```python
from build123d import *

# Parameters (mm, degrees)
SKETCH1_R           = 1.7907
SKETCH1_R_2         = 2.2987
BOSS_EXTRUDE1_DEPTH = 6.35
FILLET1_R           = 2.54
SKETCH2_W           = 2.54
SKETCH2_H           = 12.7
CUT_EXTRUDE1_DEPTH  = 6.35


with BuildPart() as part:
    # Sketch1 → Boss-Extrude1 (new body)
    with BuildSketch(Plane(origin=(0, 0, 0), x_dir=(1, 0, 0), z_dir=(0, 1, 0))):
        with BuildLine():
            Line((-12.7, -8.1407), (12.7, -8.1407))
            Line((12.7, -8.1407), (7.941309086, -1.7907))
            ThreePointArc((7.941309086, -1.7907), (7.76561659, 2.442579676), (5.48636952, 6.014212))
            ThreePointArc((5.48636952, 6.014212), (0, 21.3487), (-5.48636952, 6.014212))
            ThreePointArc((-5.48636952, 6.014212), (-7.76561659, 2.442579676), (-7.941309086, -1.7907))
            Line((-7.941309086, -1.7907), (-12.7, -8.1407))
        make_face()
        Circle(SKETCH1_R, mode=Mode.SUBTRACT)
        with Locations((0, 12.7)):
            Circle(SKETCH1_R_2, mode=Mode.SUBTRACT)
    extrude(amount=BOSS_EXTRUDE1_DEPTH)

    # Fillet1
    fillet1_edges = [part.edges().sort_by_distance(p)[0] for p in [
        (-7.941309086, 3.175, 1.7907),
        (-5.48636952, 3.175, -6.014212),
        (5.48636952, 3.175, -6.014212),
        (7.941309086, 3.175, 1.7907),
        (12.7, 3.175, 8.1407),
        (-12.7, 3.175, 8.1407),
    ]]
    fillet(fillet1_edges, radius=FILLET1_R)

    # Sketch2 → Cut-Extrude1 (cut)
    with BuildSketch(Plane(origin=(0, 6.35, 0), x_dir=(1, 0, 0), z_dir=(0, 1, 0))):
        with Locations((0, 12.7)):
            Rectangle(SKETCH2_W, SKETCH2_H)
    extrude(amount=-CUT_EXTRUDE1_DEPTH, mode=Mode.SUBTRACT)


solid = part.part
```
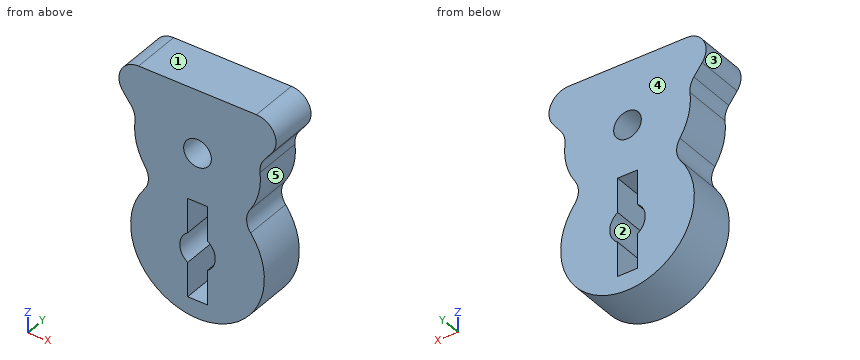
Source: CAD feature listing. Evaluate the final solid. Frame: model axes, mm. Face numbers are marked on the shaded views. A direction names the side the tool comes from. Coordinates: 2 decimals unless noted, no trailing zeros. Loops run counter-clockwise (first coordinate to the right, second up) from the corner with the lowest first, then second, coordinate; pieces in that order, holes last. Notation, with made-up numbers: (34, -22.75) -> (89, -22.75) arc R18 cw to (89, 0.25) -> close; hole circle Ø9 at (19.25, 28). An arc over 180 degrees is marked (long way). One line per item, written item: value. Start each with the question number.
Q1. Section query C-C, the plane z = -18.25. Return the cut outline in (x, y), and give its area (3 significant figures).
Q2. Section query D-D, the plane y = 5.5. Give the number of separate pieces and of enclosed holes in the cut face, and give its area (3 significant figures).
Q3. Section query A-A, the plane z = -12.7. Return the cut outline in (x, y), and give its area (3 significant figures).
Q4. Section query B-B, the plane x = 0. Return the cut outline in (y, z).
Q5. Mould query, pull axis Z, two halves, no side actions, for the marked faces 3, 4 and 5. Classes: pulls with the +Z half, pulls with the -Z half, needs draft (parallel to the pull), parting line crosses it, or undercut.
Q6. Contact query for flat-ended pins moving along their axis: P1, Ø2, axis at x = 7, y = 1, coming from the -Z side; P2, Ø2, axis at y = 5.5, z = -12, coming from the +X side; P3, Ø2, axis at y = 3, z = -9, coming from the +X side; P4, Ø2, axis at x = 0, z = 0, coming from the +Y side. Output: stop coordinate, or through.
Q7. Line query: line 1 along Z through (x, y) = (0, 4.25); line 2 along X through (y, z) = (2.5, 0); line 3 along Z through (x, y) = (-7, 5.5). Output: solid intervals per line, ascending.
Q8. Set-up query: the marked faces 1 and 2. Return all of +Z, -Z, +X, -X, +Y, -Y with unobstructed straight access to the full face (end or side cutting, diameter ignored); none if empty.
Results:
1. outline: (-6.63, 0) -> (-1.27, 0) -> (-1.27, 6.35) -> (-6.63, 6.35) -> close; (1.27, 0) -> (6.63, 0) -> (6.63, 6.35) -> (1.27, 6.35) -> close
1. area: 68.1 mm^2
2. separate pieces: 1
2. enclosed holes: 2
2. area: 411 mm^2
3. outline: (-8.65, 0) -> (-2.3, 0) -> (-2.3, 6.35) -> (-8.65, 6.35) -> close; (2.3, 0) -> (8.65, 0) -> (8.65, 6.35) -> (2.3, 6.35) -> close
3. area: 80.6 mm^2
4. outline: (0, -21.35) -> (6.35, -21.35) -> (6.35, -19.05) -> (0, -19.05) -> close; (0, -6.35) -> (6.35, -6.35) -> (6.35, -1.79) -> (0, -1.79) -> close; (0, 1.79) -> (6.35, 1.79) -> (6.35, 8.14) -> (0, 8.14) -> close
5. face 3: parting line crosses it
5. face 4: needs draft
5. face 5: undercut
6. P1: z = -18.93
6. P2: x = 8.65
6. P3: x = 8.22
6. P4: through
7. line 1: -21.35 to -19.05, -6.35 to -1.79, 1.79 to 8.14
7. line 2: -8.14 to -1.79, 1.79 to 8.14
7. line 3: -17.78 to -7.62, -4.16 to 8.14
8. face 1: +Z, +X, -X, +Y, -Y
8. face 2: +Y, -Y
